The listing builds one solid part. Answer for the finished solid, in the listing's coordinates (mm). Coordinates: 2 decimals unless noted, no trailing zeros. Write each loop counter-clockwise with the first axis right and the second up, starting at its lowest first coordinate (ties: lowest second). Pieces come first, ordered by that corner, then holes. Notation, with made-up numbers: M 23.5,-27.5 L 70.5,-27.5 A9 ccw 70.5,-11.5 Z; hole C 36,-2 d11. An arc over 180 degrees is marked long. Put each result on its own line as item: value. Start each with the question number.
```python
from build123d import *

# Parameters (mm, degrees)
KNIT_START       = -93
KNIT_1_OUTLINE_R = 62.02666435
KNIT_1_DEPTH     = 186


# Read off the part's stored shape, not the designer's step: 曲面-缝合1
with BuildPart() as part:
    # Knit 1 outline → Knit 1 (new body)
    with BuildSketch(Plane.XY.offset(KNIT_START)):
        Circle(KNIT_1_OUTLINE_R)
    extrude(amount=KNIT_1_DEPTH)


solid = part.part
```
1) A cutting plane is placed at A-A on z = 76. Write down the section's boundary in (x, y).
2) A cutting plane is placed at C-C on y = 52. Write down the section's boundary in (x, z).
3) Given pin 1 Ø6 at (x, z) = (-38, -59) entering from +Y; pin 2 Ø6 at (x, z) = (-14.5, 47.5) entering from -Y; pin 3 Ø1 at (x, z) = (45.5, -54.5) entering from -Y, each flat-ended and moving along its own axis, determine where each tip first touches the part or whether it passes through.
4) A cutting plane is placed at B-B on x = -33.5. Write down the section's boundary in (y, z), then the cut area to 3 significant figures.
5) Straight lines are drawn through the part: probe 1 along Y at (x, z) = (-45.5, -72.5); probe 2 along Y at (x, z) = (-3, -82.5); probe 3 along X at (y, z) = (19.5, 12). For each, find the intervals that lie inside material, in ascending order.
Answers follow:
1. outline: C 0,0 d124.05
2. outline: M -33.81,-93 L 33.81,-93 L 33.81,93 L -33.81,93 Z
3. pin 1: stops at y = 51.21
3. pin 2: stops at y = -60.95
3. pin 3: stops at y = -42.69
4. outline: M -52.2,-93 L 52.2,-93 L 52.2,93 L -52.2,93 Z
4. area: 19,400 mm²
5. probe 1: y = -42.16 to 42.16
5. probe 2: y = -61.95 to 61.95
5. probe 3: x = -58.88 to 58.88
